Input: part model. Units: mm. Frame: model coordinates. A direction names the side the tool comes from. Round coordinates to 2 decimals unless told otherwise and drop trailing zeros. Loops run counter-clockwise (first coordinate to the right, second up) from the corner with the lowest first, then second, coordinate; pieces in that order, holes last.
(1) Draft query along X for faces 1 (the face through (88, 40.64, 3)), 2 (the face through (138.39, 29.3, 2.98)), 3 (the face through (7.127, 53.505, 2.98)), 4 (the face through (49, 38, 6.045)). Return one class per face: released by +X, released by -X, zero draft, split by the parting line, or undercut.
(2) Cut plane B-B, the plane x = 67. Output: boundary loops of the cut face in (y, z) (3 decimals).
(3) First-contact query: pin 1 Ø3 at (x, z) = (104.5, 4.5) entering from -Y (3 decimals); pin 2 Ø5.5 at (x, y) = (0, 0) entering from -Z; pin 3 Ø3 at (y, z) = (45, 3) entering from -X. Flat tips, straight axial feed; report the tip coordinate or a pass-through.
(4) Cut plane A-A, the plane z = 2. Give the number of separate pieces and of enclosed holes in the cut face, and give its area (3 significant figures).
(5) Line query: line 1 (Y direction, x = 44.5, z = 4.5) (3 decimals); line 2 (X direction, y = 41.5, z = 2.75); line 3 (X direction, y = 43.5, z = 2.5). Output: solid intervals per line, ascending.
(6) Access query for faces 5 (the face through (0.34, 47.42, 2.98)), 6 (the face through (134.393, 44, 3)). Directions: +Z, -Z, +X, -X, +Y, -Y. A direction counts if a zero-diameter tool reaches every point of the face in a straight line with its end or side. Return the directions, or none.
from build123d import *

# Parameters (mm, degrees)
SKETCH1_R           = 3.175
BOSS_EXTRUDE1_DEPTH = 6.0452
SKETCH2_W           = 15.875
SKETCH2_H           = 6.35
CUT_EXTRUDE1_DEPTH  = 6.0452


with BuildPart() as part:
    # Sketch1 → Boss-Extrude1 (new body)
    with BuildSketch(Plane.XY):
        with BuildLine():
            Line((-6.35, 38.1), (-6.35, 0))
            ThreePointArc((-6.35, 0), (-2.430039796, -5.866635031), (4.490128061, -4.490128061))
            Line((4.490128061, -4.490128061), (31.430896424, 22.450640303))
            Line((31.430896424, 22.450640303), (36.811307345, 27.831051224))
            ThreePointArc((36.811307345, 27.831051224), (37.635342651, 28.381654013), (38.607358569, 28.575))
            Line((38.607358569, 28.575), (136.615256121, 28.575))
            ThreePointArc((136.615256121, 28.575), (138.411307345, 29.318948776), (139.155256121, 31.115))
            Line((139.155256121, 31.115), (139.155256121, 51.435))
            ThreePointArc((139.155256121, 51.435), (138.411307345, 53.231051224), (136.615256121, 53.975))
            Line((136.615256121, 53.975), (9.525, 53.975))
            ThreePointArc((9.525, 53.975), (7.094960204, 53.491635031), (5.034871939, 52.115128061))
            Line((5.034871939, 52.115128061), (-4.490128061, 42.590128061))
            ThreePointArc((-4.490128061, 42.590128061), (-5.866635031, 40.530039796), (-6.35, 38.1))
        make_face()
        Circle(SKETCH1_R, mode=Mode.SUBTRACT)
        with BuildLine():
            ThreePointArc((25.818236348, 25.818236348), (13.972728824, 33.733151431), (0, 36.5125))
            ThreePointArc((0, 36.5125), (-1.5875, 38.1), (0, 39.6875))
            ThreePointArc((0, 39.6875), (15.187748722, 36.666468947), (28.063300378, 28.063300378))
            ThreePointArc((28.063300378, 28.063300378), (28.063300378, 25.818236348), (25.818236348, 25.818236348))
        make_face(mode=Mode.SUBTRACT)
    extrude(amount=BOSS_EXTRUDE1_DEPTH)

    # Sketch2 → Cut-Extrude1 (cut)
    with BuildSketch(Plane.XY.offset(6.0452)):
        with Locations((126.455256121, 43.815)):
            Rectangle(SKETCH2_W, SKETCH2_H)
        with Locations((88.355256121, 43.815)):
            Rectangle(SKETCH2_W, SKETCH2_H)
        with Locations((50.255256121, 43.815)):
            Rectangle(SKETCH2_W, SKETCH2_H)
    extrude(amount=-CUT_EXTRUDE1_DEPTH, mode=Mode.SUBTRACT)


solid = part.part
Reported:
1. face 1: undercut
1. face 2: released by +X
1. face 3: released by -X
1. face 4: zero draft
2. outline: (28.575, 0) - (53.975, 0) - (53.975, 6.045) - (28.575, 6.045) - close
3. pin 1: stops at y = 28.575
3. pin 2: passes through
3. pin 3: stops at x = -3.58
4. separate pieces: 1
4. enclosed holes: 5
4. area: 4,080 mm2
5. line 1: y = 28.575 to 40.64, 46.99 to 53.975
5. line 2: x = -5.36 to 42.32, 58.19 to 80.42, 96.29 to 118.52, 134.39 to 139.16
5. line 3: x = -3.58 to 42.32, 58.19 to 80.42, 96.29 to 118.52, 134.39 to 139.16
6. face 5: +Z, -Z, -X, +Y
6. face 6: +Z, -Z
